Verification items for the finished model (mm, model axes). Coordinates: 2 decimals unless noted, no trailing zeros. Order: outer loops, then holes, each group sorted by start corner. A loop starts at its lowest first (then second) coordinate and runs counter-clockwise, first axis right, second up. Notation, with made-up numbers: (16, 87) -> (26, 87) arc R19 cw to (26, 119) -> close; hole circle Ø7 at (20, 33.25). An arc over 180 degrees is marked (long way). Write each question's results on one line, items separated by ' | '. Start each with the question number.
(1) Cross-section at A-A on x = -379. Enter the section's corners in (y, z).
(2) Go/stop test with flat-tipped pins: pin 1 (2 mm diameter, centred on x = -468.5, z = 53.5, fed in from -Y); pin 2 (12 mm diameter, centred on x = -866.5, z = -57.5, fed in from +Y). Record where each tip stops, or that it passes through.
(3) Thickness scan on probe 1 along Y at (x, z) = (-287.5, -17); probe 2 along Y at (x, z) = (-858.5, -2.5); probe 3 along Z at (x, y) = (-862, 1671). Record the ranges inside material, lowest first. Write a range as [from, to].
(4) Cross-section at B-B on y = 1639.5. Enter the section's corners in (x, z).
```python
from build123d import *

# Parameters (mm, degrees)
BOSS_EXTRUDE1_DEPTH      = 508
BOSS_EXTRUDE1_DEPTH_BACK = 508
CUT_EXTRUDE2_DEPTH       = 1961.143295518
CUT_EXTRUDE2_DEPTH_BACK  = 1961.143295518
CUT_EXTRUDE7_DEPTH       = 2719.400028326
CUT_EXTRUDE7_DEPTH_BACK  = 2719.400028326


with BuildPart() as part:
    # Sketch1 → Boss-Extrude1 (new, two sides: drawn at the far end of the back side and taken through both)
    with BuildSketch(Plane(origin=(0, 0, 0), x_dir=(0, 1, 0), z_dir=(0, 0, 1)).offset(-BOSS_EXTRUDE1_DEPTH_BACK)):
        Polygon((0, 0), (1219.2, 989.685264987), (2438.4, 0), (1473.631984251, 1194.282750762), (964.768015749, 1194.282750762), align=None)
    extrude(amount=BOSS_EXTRUDE1_DEPTH + BOSS_EXTRUDE1_DEPTH_BACK)

    # Sketch2 → Cut-Extrude2 (cut, two sides: drawn at the far end of the back side and taken through both)
    with BuildSketch(Plane(origin=(-1193.155493259, 968.543643797, 0), x_dir=(0.6302416824749717, 0.7763990093187376, 0), z_dir=(0.7763990093187376, -0.6302416824749717, 0)).offset(-CUT_EXTRUDE2_DEPTH_BACK)):
        Polygon((1893.171344323, -508), (1893.171344323, 0), (-138.828655677, -142.091281869), (-138.828655677, -508), align=None)
        Polygon((-138.828655677, 142.091281869), (1893.171344323, 0), (1893.171344323, 508), (-138.828655677, 508), align=None)
    extrude(amount=CUT_EXTRUDE2_DEPTH + CUT_EXTRUDE2_DEPTH_BACK, mode=Mode.SUBTRACT)

    # Sketch5 → Cut-Extrude7 (cut, two sides: drawn at the far end of the back side and taken through both)
    with BuildSketch(Plane(origin=(0, 0, 0), x_dir=(0, 1, 0), z_dir=(0, 0, 1)).offset(-CUT_EXTRUDE7_DEPTH_BACK)):
        Polygon((2438.4, 0), (965.713353388, 1195.452980721), (0, 0), align=None)
    extrude(amount=CUT_EXTRUDE7_DEPTH + CUT_EXTRUDE7_DEPTH_BACK, mode=Mode.SUBTRACT)


solid = part.part
```
Results are:
1) outline: (1971.51, -42.05) -> (2132.24, -33.32) -> (2132.24, 33.32) -> (1971.51, 42.05) -> close
2) pin 1: passes through | pin 2: stops at y = 1743.27
3) probe 1: y = [2084.23, 2206.15] | probe 2: y = [1380.81, 1744.88] | probe 3: z = [-79.65, 79.65]
4) outline: (-988.96, -86.96) -> (-648.51, -71.95) -> (-648.51, 71.95) -> (-988.96, 86.96) -> close
